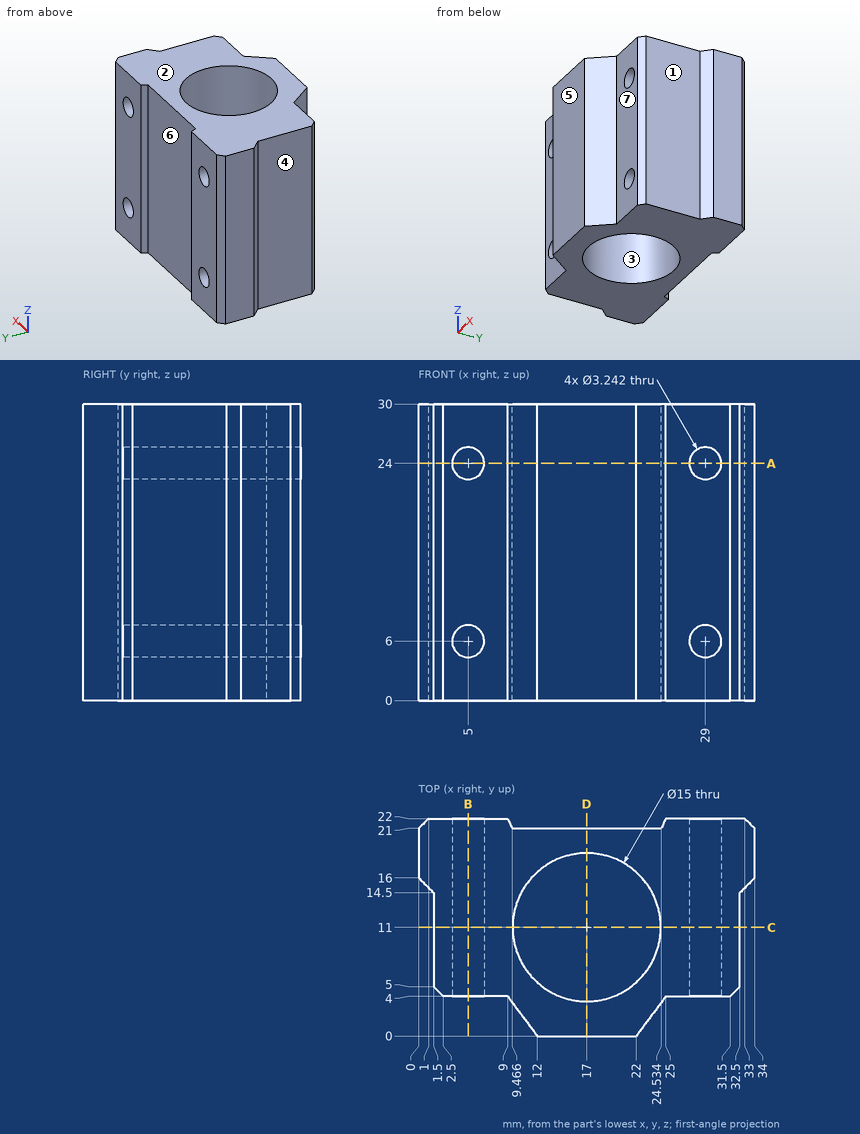
Geometry check sheet. Reference: drawing and pictorial views, mm from the part's lowest x, y, z. A direction names the side the tool comes from. Coordinates: 2 decimals unless noted, no trailing zeros. Order: outer loops, then holes, each group sorted by start corner. A loop starts at its lowest first (then second) coordinate and runs counter-clockwise, first axis right, second up.
Item 1: Section check D-D (x = 17). Enter the section's corners in (y, z).
Item 2: Mould release check, pull along X, two halves, no side actions. Record for the marked faces 1, 2 and 3: released by +X, released by -X, zero draft, split by the parting line, or undercut.
Item 3: Scan lines: line 1 along Z through (x, y) = (29, 14.5); line 2 along X through (y, z) = (19.5, 24); line 3 along X through (y, z) = (17.5, 6). Record each from-to range of solid material in increasing order.
Item 4: Depth check by flat-ended pin: pin 1 (3 mm diameter, centred on x = 12.5, z = 20, fed in from +Y); pin 2 (7.5 mm diameter, centred on y = 8, z = 15.5, fed in from -X); pin 3 (2 mm diameter, centred on x = 6, z = 19, fed in from -Y); pin 4 (3 mm diameter, centred on x = 5, z = 24, fed in from +Y). Enter the tip coordinate at first touch or a pass-through.
Item 5: Section check C-C (y = 11). Enter the section's corners in (x, z), plus the area to 3 significant figures.
Item 6: Tool access check on the marked faces 4, 5, 6 and 7. Record the directions out of +Z, -Z, +X, -X, +Y, -Y that give a thin tool (end or side, any length) a straight path to the whole face; none if there is none.
Item 7: Section check A-A (z = 24). Count the separate pieces of the cut face and the enclosed holes in it, plus the area to 3 significant figures.
Item 8: Section check B-B (x = 5). Enter the section's corners in (y, z).
Check sheet entries:
1. outline: (0, 0) - (3.5, 0) - (3.5, 30) - (0, 30) - close; (18.5, 0) - (21, 0) - (21, 30) - (18.5, 30) - close
2. face 1: released by +X
2. face 2: zero draft
2. face 3: undercut
3. line 1: z = 0 to 4.38, 7.62 to 22.38, 25.62 to 30
3. line 2: x = 0 to 3.38, 6.62 to 27.38, 30.62 to 34
3. line 3: x = 0 to 3.38, 6.62 to 13.26, 20.74 to 27.38, 30.62 to 34
4. pin 1: stops at y = 21
4. pin 2: stops at x = 1.5
4. pin 3: stops at y = 4
4. pin 4: passes through
5. outline: (1.5, 0) - (9.5, 0) - (9.5, 30) - (1.5, 30) - close; (24.5, 0) - (32.5, 0) - (32.5, 30) - (24.5, 30) - close; hole circle Ø3.24 at (5, 6); hole circle Ø3.24 at (5, 24); hole circle Ø3.24 at (29, 6); hole circle Ø3.24 at (29, 24)
5. area: 447 mm2
6. face 4: +Z, -Z, -X, -Y
6. face 5: +Z, -Z, +X, -X, -Y
6. face 6: +Z, -Z, +Y
6. face 7: +Z, -Z, +X, -Y
7. separate pieces: 3
7. enclosed holes: 1
7. area: 319 mm2
8. outline: (4, 0) - (22, 0) - (22, 4.38) - (4, 4.38) - close; (4, 7.62) - (22, 7.62) - (22, 22.38) - (4, 22.38) - close; (4, 25.62) - (22, 25.62) - (22, 30) - (4, 30) - close
